from build123d import *

# Parameters (mm, degrees)
BOSS_EXTRUDE1_DEPTH = 7
SKETCH2_R           = 8.5
BOSS_EXTRUDE2_DEPTH = 7
SKETCH3_R           = 6.51
CUT_EXTRUDE1_DEPTH  = 5
SKETCH4_R           = 4
CUT_EXTRUDE2_DEPTH  = 72.699089491
SKETCH5_R           = 6
CUT_EXTRUDE3_DEPTH  = 72.866260748


with BuildPart() as part:
    # Sketch1 → Boss-Extrude1 (new body)
    with BuildSketch(Plane.XY):
        Polygon((0, 0), (45, 0), (22.5, 38.97114317), align=None)
    extrude(amount=BOSS_EXTRUDE1_DEPTH)

    # Sketch2 → Boss-Extrude2 (add)
    with BuildSketch(Plane.XY.offset(7)):
        Circle(SKETCH2_R)
        with Locations((45, 0)):
            Circle(SKETCH2_R)
        with Locations((22.5, 38.97114317)):
            Circle(SKETCH2_R)
    extrude(amount=-BOSS_EXTRUDE2_DEPTH)

    # Sketch3 → Cut-Extrude1 (cut)
    with BuildSketch(Plane.XY.offset(7)):
        Circle(SKETCH3_R)
        with Locations(Location((45, 0, 0), (0, 0, 180))):
            Circle(SKETCH3_R)
        with Locations((22.5, 38.97114317)):
            Circle(SKETCH3_R)
    extrude(amount=-CUT_EXTRUDE1_DEPTH, mode=Mode.SUBTRACT)

    # Sketch4 → Cut-Extrude2 (cut, through all)
    with BuildSketch(Plane.XY.offset(2)):
        Circle(SKETCH4_R)
        with Locations(Location((45, 0, 0), (0, 0, 180))):
            Circle(SKETCH4_R)
        with Locations((22.5, 38.97114317)):
            Circle(SKETCH4_R)
    extrude(amount=-CUT_EXTRUDE2_DEPTH, mode=Mode.SUBTRACT)

    # Sketch5 → Cut-Extrude3 (cut, through all)
    with BuildSketch(Plane.XY.offset(7)):
        with Locations((22.5, 12.990381057)):
            Circle(SKETCH5_R)
    extrude(amount=-CUT_EXTRUDE3_DEPTH, mode=Mode.SUBTRACT)


solid = part.part
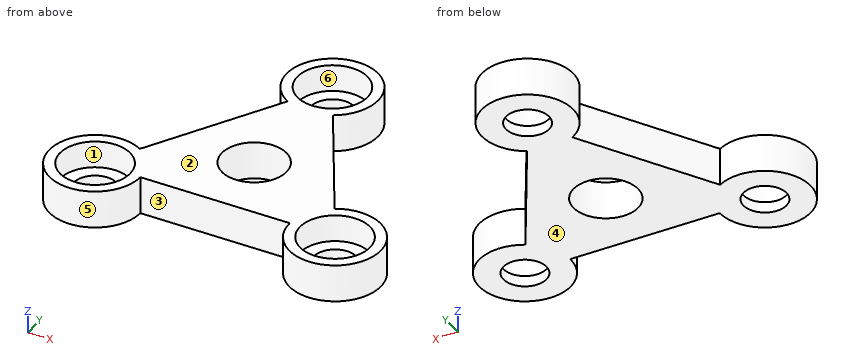
For this review, take the finished solid that the model builds, in its own axes (mm). Face numbers are marked on the shaded views. A direction names the side the tool comes from. Give positions to 0.01 mm unless a question says otherwise; leave off trailing zeros. Order: outer loops, then holes, each group sorted by start corner. A loop starts at its lowest first (then second) coordinate and runs counter-clockwise, first axis right, second up. Notation, with made-up numbers: (2, 1.5) - (19, 1.5) arc R15 cw to (19, 22.5) - close; hole circle Ø9 at (9.5, 12). An arc over 180 degrees is marked (long way). Answer as a JSON object with one key per item and string values. Group by question number.
Item 1: Draft analysis for pull direction Y (two halves, no side actions). For the marked faces 3, 4, 5 and 6, state which applies: pulls with the +Y half, pulls with the -Y half, needs draft (parallel to the pull), parting line crosses it, or undercut.
Item 2: Clearance check with flat-ended pins moving along their axes: pin 1 Ø10.5 at (x, y) = (45, 0) entering from +Z; pin 2 Ø7 at (x, y) = (0, 0) entering from +Z; pin 3 Ø6.5 at (x, y) = (19.5, 36) entering from +Z; pin 4 Ø4 at (x, z) = (31.5, 4) entering from +Y. State where each tip first meets the part, or that it passes through.
Item 3: Take a section at A-A on x = 48. Give the boundary of the cut face in (y, z).
Item 4: Machinability: for the marked faces 1 and 2, which of the approach directions +Z, -Z, +X, -X, +Y, -Y give a long, thin tool a straight path to every point of the face, cutting with its end or side? Answer none if there is none.
Item 5: Take a section at C-C on y = 10.5. Give the boundary of the cut face in (x, z).
Item 6: Wall thickness on line 1 along Y through (x, z) = (24, 5.75); line 2 along Y through (x, z) = (0, 1.35); line 3 along Y through (x, z) = (26, 5.25): over which ranges is each line inside the solid? List them lowest first.
Item 7: Take a section at B-B on x = 22.5. Give the boundary of the cut face in (y, z), and give its area (3 significant figures).
Item 8: Take a section at D-D on z = 3. Give the boundary of the cut face in (x, y).
Reported:
{
 "1": {"face 3": "pulls with the -Y half", "face 4": "needs draft", "face 5": "parting line crosses it", "face 6": "undercut"},
 "2": {"pin 1": "z = 2", "pin 2": "through", "pin 3": "z = 7", "pin 4": "y = 43.79"},
 "3": {"outline": "(-7.95, 0) - (-2.65, 0) - (-2.65, 2) - (-5.78, 2) - (-5.78, 7) - (-7.95, 7) - close; (2.65, 0) - (7.95, 0) - (7.95, 7) - (5.78, 7) - (5.78, 2) - (2.65, 2) - close"},
 "4": {"face 1": "+Z", "face 2": "+Z, +X, -X, +Y, -Y"},
 "5": {"outline": "(6.06, 0) - (17.04, 0) - (17.04, 7) - (6.06, 7) - close; (27.96, 0) - (38.94, 0) - (38.94, 7) - (27.96, 7) - close"},
 "6": {"line 1": "0 to 7.18, 18.8 to 32.64, 45.31 to 47.34", "line 2": "-8.5 to -4, 4 to 8.5", "line 3": "0 to 8.12, 17.86 to 33.48, 44.46 to 46.72"},
 "7": {"outline": "(0, 0) - (6.99, 0) - (6.99, 7) - (0, 7) - close; (18.99, 0) - (34.97, 0) - (34.97, 2) - (32.46, 2) - (32.46, 7) - (18.99, 7) - close; (42.97, 0) - (47.47, 0) - (47.47, 7) - (45.48, 7) - (45.48, 2) - (42.97, 2) - close", "area": "167 mm^2"},
 "8": {"outline": "(4.25, 7.36) arc R8.5 ccw (long way) to (8.5, 0) - (36.5, 0) arc R8.5 ccw (long way) to (40.75, 7.36) - (26.75, 31.61) arc R8.5 ccw (long way) to (18.25, 31.61) - close; hole circle Ø13.02 at (0, 0); hole circle Ø13.02 at (22.5, 38.97); hole circle Ø12 at (22.5, 12.99); hole circle Ø13.02 at (45, 0)"}
}
